The listing builds one solid part. Answer for the finished solid, in the listing's coordinates (mm). A direction names the side the tool comes from. Round coordinates to 2 decimals unless told otherwise and drop trailing zeros. Write each loop counter-clockwise with the first axis right and the second up, starting at its lowest first coordinate (ties: lowest second). Pieces come first, ordered by that corner, then holes.
(1) Find the intervals of material crossed by probe 1 along Z at (x, y) = (0, -10); probe 2 along Z at (x, y) = (0, -0.35); probe 3 along X at (y, z) = (-17.75, 77.5), in increasing order.
(2) For faces 1 (the face through (-0.65, -11.35, 72.07)), 2 (the face through (1, -22, 78)), determine the directions among +Z, -Z, +X, -X, +Y, -Y from which every point of the face is accessible in a straight line to the end or side of a thin tool.
(3) A cutting plane is placed at B-B, the plane x = 0. Give the vertices of the cut face in (y, z).
(4) A cutting plane is placed at C-C, the plane y = -5. Give the vertices of the cut face in (x, z), and give its area (3 significant figures).
(5) A cutting plane is placed at D-D, the plane x = -2.75. Give the vertices of the cut face in (y, z), and give its area (3 significant figures).
(6) The mould has two halves that part along X. Classify faces 3 (the face through (-0.867, -10.846, 71.095)), 4 (the face through (1.3, -1, 75)), 5 (the face through (1, 0, 74)): +X half, -X half, draft (parallel to the pull), parting line (faces both ways), or undercut.
(7) Each of these flat-tipped pins is pushed along its axis until it touches: pin 1 Ø1.5 at (y, z) = (-8.5, 74.5) entering from -X; pin 2 Ø1.5 at (x, z) = (0, 73.5) entering from -Y. Where does it stop, or does it pass through?
(8) A cutting plane is placed at A-A, the plane z = 75. Give the vertices of the cut face in (x, y).
from build123d import *

# Parameters (mm, degrees)
CYLINDER_R             = 3
CYLINDER_DEPTH         = 22
CYLINDER_ROLL_ANGLE    = 90
CYLINDER013_R          = 1.15
CYLINDER013_DEPTH      = 6
CYLINDER013_ROLL_ANGLE = 90
CYLINDER010_R          = 4
CYLINDER010_DEPTH      = 22
CYLINDER010_ROLL_ANGLE = 90


with BuildPart() as cylinder:
    # Cylinder → Cylinder (new body)
    with BuildSketch(Plane.XY):
        Circle(CYLINDER_R)
    extrude(amount=CYLINDER_DEPTH)


with BuildPart() as cylinder_1:
    # Cylinder roll: moved
    add(cylinder.part.rotate(Axis((0, 0, 0), (1, 0, 0)), CYLINDER_ROLL_ANGLE))


with BuildPart() as cylinder_2:
    # Cylinder placement: moved
    add(cylinder_1.part.moved(Location((0, -1, 75))))


with BuildPart() as fusion:
    # Cylinder013 → Cylinder013 (new body)
    with BuildSketch(Plane.XY):
        Circle(CYLINDER013_R)
    extrude(amount=CYLINDER013_DEPTH)


with BuildPart() as fusion_1:
    # Cylinder013 roll: moved
    add(fusion.part.rotate(Axis((0, 0, 0), (1, 0, 0)), CYLINDER013_ROLL_ANGLE))


with BuildPart() as fusion_2:
    # Cylinder013 placement: moved
    add(fusion_1.part.moved(Location((0, 5, 75))))

    # Fusion: union Cylinder
    add(cylinder_2.part)


with BuildPart() as cut002:
    # Cylinder010 → Cylinder010 (new body)
    with BuildSketch(Plane.XY):
        Circle(CYLINDER010_R)
    extrude(amount=CYLINDER010_DEPTH)


with BuildPart() as cut002_1:
    # Cylinder010 roll: moved
    add(cut002.part.rotate(Axis((0, 0, 0), (1, 0, 0)), CYLINDER010_ROLL_ANGLE))


with BuildPart() as cut002_2:
    # Cylinder010 placement: moved
    add(cut002_1.part.moved(Location((0, 0, 75))))

    # Cut002: cut Fusion
    add(fusion_2.part, mode=Mode.SUBTRACT)


solid = cut002_2.part
Solutions:
1. probe 1: z = 71 to 72, 78 to 79
1. probe 2: z = 71 to 73.85, 76.15 to 79
1. probe 3: x = -3.12 to -1.66, 1.66 to 3.12
2. face 1: -Y
2. face 2: +Z, -Z, +X, -X, -Y
3. outline: (-22, 71) - (0, 71) - (0, 73.85) - (-1, 73.85) - (-1, 72) - (-22, 72) - close; (-22, 78) - (-1, 78) - (-1, 76.15) - (0, 76.15) - (0, 79) - (-22, 79) - close
4. outline: circle Ø8 at (0, 75); hole circle Ø6 at (0, 75)
4. area: 22.0 mm2
5. outline: (-22, 72.1) - (0, 72.1) - (0, 77.9) - (-22, 77.9) - (-22, 76.2) - (-1, 76.2) - (-1, 73.8) - (-22, 73.8) - close
5. area: 77.5 mm2
6. face 3: parting line
6. face 4: undercut
6. face 5: draft
7. pin 1: stops at x = -4
7. pin 2: stops at y = -1
8. outline: (-4, -22) - (-3, -22) - (-3, -1) - (-1.15, -1) - (-1.15, 0) - (-4, 0) - close; (1.15, -1) - (3, -1) - (3, -22) - (4, -22) - (4, 0) - (1.15, 0) - close
